Check sheet for the modelled part. Datum: model origin and axes. Units: mm. Round coordinates to 2 decimals unless told otherwise and drop trailing zeros. Write each loop counter-clockwise with the first axis right and the second up, starting at its lowest first coordinate (ties: lowest second). Pieces come first, ordered by that corner, then holes. Notation, with made-up numbers: M 73,84.25 L 84,84.25 A26 ccw 84,98.25 Z; hole C 88,36.25 d1. An arc over 180 degrees is marked long. Answer in a Markdown table with one row per item.
```python
from build123d import *

# Parameters (mm, degrees)
CROQUIS1_W              = 180
CROQUIS1_H              = 230
CROQUIS1_R              = 2.5
SALIENTE_EXTRUIR1_DEPTH = 3


with BuildPart() as part:
    # Croquis1 → Saliente-Extruir1 (new body)
    with BuildSketch(Plane.XY):
        with Locations((90, -115)):
            Rectangle(CROQUIS1_W, CROQUIS1_H)
        with Locations((175.5, -115)):
            Circle(CROQUIS1_R, mode=Mode.SUBTRACT)
        Polygon((90, -56.5), (136.5, -56.5), (136.5, -173.5), (43.5, -173.5), (43.5, -56.5), align=None, mode=Mode.SUBTRACT)
    extrude(amount=SALIENTE_EXTRUIR1_DEPTH)


solid = part.part
```
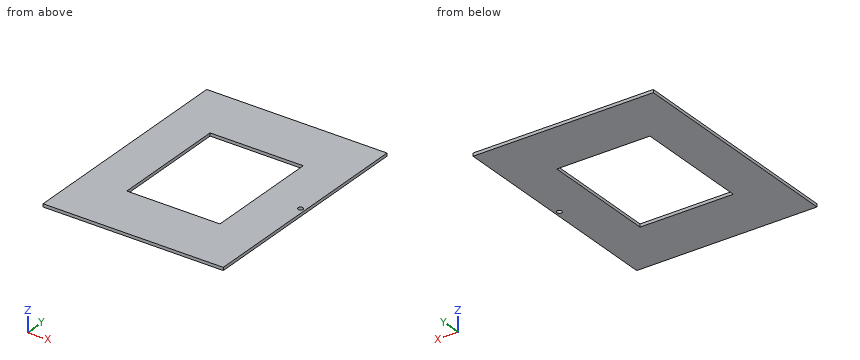
1. Section check C-C, the plane z = 1.95. Record the cut outline in (x, y).
Found:
| item | result |
|---|---|
| outline | M 0,-230 L 180,-230 L 180,0 L 0,0 Z; hole M 43.5,-173.5 L 136.5,-173.5 L 136.5,-56.5 L 43.5,-56.5 Z; hole C 175.5,-115 d5 |
2. Section check A-A, the plane x = 175.5. Record the cut outline in (y, z), and give its area (3 significant figures).
Found:
| item | result |
|---|---|
| outline | M -230,0 L -117.5,0 L -117.5,3 L -230,3 Z; M -112.5,0 L 0,0 L 0,3 L -112.5,3 Z |
| area | 675 mm2 |
3. Scan lines: L1, parallel to Y at x = 115, z = 1.2; L2, parallel to X at y = -168, z = 1.75; L3, parallel to Y at x = 175.5, z = 0.7. Record each from-to range of solid material in increasing order.
Found:
| item | result |
|---|---|
| L1 | y = -230 to -173.5, -56.5 to 0 |
| L2 | x = 0 to 43.5, 136.5 to 180 |
| L3 | y = -230 to -117.5, -112.5 to 0 |
4. Section check B-B, the plane y = -115. Record the cut outline in (x, z).
Found:
| item | result |
|---|---|
| outline | M 0,0 L 43.5,0 L 43.5,3 L 0,3 Z; M 136.5,0 L 173,0 L 173,3 L 136.5,3 Z; M 178,0 L 180,0 L 180,3 L 178,3 Z |
